Autodesk Inventor part; units mm, degrees
ref_plane "YZ Plane" through (0, 0, 0) normal (1, 0, 0) x (0, 1, 0)
ref_plane "XZ Plane" through (0, 0, 0) normal (0, 1, 0) x (-1, 0, 0)
ref_plane "XY Plane" through (0, 0, 0) normal (0, 0, 1) x (1, 0, 0)
sketch "Sketch1" plane through (0, 0, 0) normal (0, 0, 1) x (1, 0, 0)
  line L0 (-20, -12.5) -> (20, -12.5)
  line L1 (20, -12.5) -> (20, 12.5)
  line L2 (20, 12.5) -> (-20, 12.5)
  line L3 (-20, 12.5) -> (-20, -12.5)
  line L4 (-20, -12.5) -> (20, 12.5) construction
  line L5 (20, -12.5) -> (-20, 12.5) construction
  point P0 (0, 0)
  dimension "d0" = 40
  dimension "d1" = 25
extrude "Extrusion1" add sketch "Sketch1" against normal blind 15
sketch "Sketch2" plane through (0, 0, 0) normal (0, 0, 1) x (1, 0, 0)
  line L0 (20, 12.5) -> (20, -12.5)
  line L1 (20, 12.5) -> (5, 12.5)
  line L2 (5, 12.5) -> (5, -2.5)
  line L3 (5, -2.5) -> (20, -2.5)
  line L4 (20, -2.5) -> (20, 12.5)
  point P0 (0, 0)
  dimension "d4" = 15
  dimension "d5" = 15
extrude "Extrusion2" cut sketch "Sketch2" against normal blind 8
properties part number "desenho 2"
Verification items for the finished model (mm, model axes). A direction names the side the tool comes from. Give positions to 0.01 mm unless a question says otherwise; leave off trailing zeros. Write each loop counter-clockwise with the first axis right and the second up, starting at its lowest first coordinate (ties: lowest second). Pieces come first, ordered by that corner, then holes. Notation, with made-up numbers: M -20,65 L 29,65 A15 cw 29,74 Z; hole C 79,89.5 d8. An arc over 180 degrees is marked long. One line per question, with ' | ' between items.
1) Section check B-B on y = 5. Enter the section's corners in (x, z).
Result:
outline: M -20,-15 L 20,-15 L 20,-8 L 5,-8 L 5,0 L -20,0 Z
2) Gauge pin test, flat end, axial feed: pin 1 Ø6.5 at (y, z) = (2.5, -4.5) entering from +X. Record the tip position at first contact, or that the pin passes through.
Result:
pin 1: stops at x = 5
3) Set-up check for faces 1 (the flat face through (-20, 0, -7)), 2 (the flat face through (12, 5, -8)): record each of +Z, -Z, +X, -X, +Y, -Y from which the full face is reachable in a straight line by a thin tool's end or side.
Result:
face 1: +Z, -Z, -X, +Y, -Y | face 2: +Z, +X, +Y
4) Thickness scan on line 1 along X through (y, z) = (5.25, -6.5); line 2 along Z through (x, y) = (10, 2); line 3 along Y through (x, z) = (7.5, -5.75). Record the ranges inside material, lowest first. Write a range as [from, to].
Result:
line 1: x = [-20, 5] | line 2: z = [-15, -8] | line 3: y = [-12.5, -2.5]
5) Section check A-A on z = -6.25. Enter the section's corners in (x, y), plus the area to 3 significant figures.
Result:
outline: M -20,-12.5 L 20,-12.5 L 20,-2.5 L 5,-2.5 L 5,12.5 L -20,12.5 Z | area: 775 mm2
